```python
from build123d import *

# Parameters (mm, degrees)
SKETCH1_R           = 17.5
BOSS_EXTRUDE1_DEPTH = 0.5
SKETCH2_R           = 11.5
CUT_EXTRUDE1_DEPTH  = 0.5
SKETCH3_W           = 15
SKETCH3_H           = 8
CUT_EXTRUDE4_DEPTH  = 2.5
SKETCH4_R           = 16
SKETCH4_R_2         = 15.5
BOSS_EXTRUDE2_DEPTH = 4.5
SKETCH5_R           = 14.5
SKETCH5_R_2         = 14
BOSS_EXTRUDE3_DEPTH = 4.5
SKETCH6_R           = 17.5
SKETCH6_R_2         = 17
BOSS_EXTRUDE4_DEPTH = 4.5


with BuildPart() as part:
    # Sketch1 → Boss-Extrude1 (new body)
    with BuildSketch(Plane(origin=(0, 0, 0), x_dir=(1, 0, 0), z_dir=(0, 1, 0))):
        with Locations(Location((0, 0, 0), (0, 0, 270))):
            Circle(SKETCH1_R)
    extrude(amount=BOSS_EXTRUDE1_DEPTH)

    # Sketch2 → Cut-Extrude1 (cut)
    with BuildSketch(Plane(origin=(0, 0.5, 0), x_dir=(1, 0, 0), z_dir=(0, 1, 0))):
        with Locations(Location((2, 0, 0), (0, 0, 270))):
            Circle(SKETCH2_R)
    extrude(amount=-CUT_EXTRUDE1_DEPTH, mode=Mode.SUBTRACT)

    # Sketch3 → Cut-Extrude4 (cut)
    with BuildSketch(Plane(origin=(0, 0, 0), x_dir=(1, 0, 0), z_dir=(0, 1, 0))):
        with Locations((-5.5, 0)):
            Rectangle(SKETCH3_W, SKETCH3_H)
    extrude(amount=CUT_EXTRUDE4_DEPTH, mode=Mode.SUBTRACT)

    # Sketch4 → Boss-Extrude2 (add)
    with BuildSketch(Plane(origin=(0, 0, 0), x_dir=(1, 0, 0), z_dir=(0, 1, 0))):
        with Locations(Location((0, 0, 0), (0, 0, 270))):
            Circle(SKETCH4_R)
        with Locations(Location((0, 0, 0), (0, 0, 270))):
            Circle(SKETCH4_R_2, mode=Mode.SUBTRACT)
    extrude(amount=BOSS_EXTRUDE2_DEPTH)

    # Sketch5 → Boss-Extrude3 (add)
    with BuildSketch(Plane(origin=(0, 0.5, 0), x_dir=(1, 0, 0), z_dir=(0, 1, 0))):
        with Locations(Location((0, 0, 0), (0, 0, 270))):
            Circle(SKETCH5_R)
        with Locations(Location((0, 0, 0), (0, 0, 270))):
            Circle(SKETCH5_R_2, mode=Mode.SUBTRACT)
    extrude(amount=BOSS_EXTRUDE3_DEPTH)

    # Sketch6 → Boss-Extrude4 (add)
    with BuildSketch(Plane(origin=(0, 0.5, 0), x_dir=(1, 0, 0), z_dir=(0, 1, 0))):
        with Locations(Location((0, 0, 0), (0, 0, 270))):
            Circle(SKETCH6_R)
        with Locations(Location((0, 0, 0), (0, 0, 270))):
            Circle(SKETCH6_R_2, mode=Mode.SUBTRACT)
    extrude(amount=BOSS_EXTRUDE4_DEPTH)


solid = part.part
```
For this review, take the finished solid that the model builds, in its own axes (mm). A direction names the side the tool comes from. Give positions to 0.01 mm unless a question says otherwise; leave off trailing zeros. Loops run counter-clockwise (first coordinate to the right, second up) from the corner with the lowest first, then second, coordinate; pieces in that order, holes last. Notation, with made-up numbers: M 83,61.25 L 94,61.25 A16 cw 94,82.25 Z; hole C 57.5,-9.75 d6. An arc over 180 degrees is marked long. One line per item, written item: value. Start each with the question number.
Q1. Draft analysis for pull direction Z (two halves, no side actions). For faces 1 (the face through (-10.648, 2.465, -13.887)), 2 (the face through (-8, 0, 8)), 3 (the face through (-13.67, 2.72, -3.03)), state which applies: released by +Z, released by -Z, zero draft, split by the parting line, or undercut.
Q2. Add section B-B (z = 0). Give the boundary of the cut face in (x, y), and give its area (4 significant figures).
Q3. For L1, parallel to X at y = 3.6, z = -4.5; L2, parallel to X at y = 3.75, z = 1, list the stretches that pass through material, from the lowest coordinate up.
Q4. Add section A-A (y = 2.8). Give the boundary of the cut face in (x, z), and give its area (3 significant figures).
Q5. Add section C-C (x = -12). Give the boundary of the cut face in (y, z), and give its area (3 significant figures).
Q6. Clearance check with flat-ended pins moving along their axes: pin 1 Ø2 at (y, z) = (1, 1.5) entering from -X; pin 2 Ø1 at (y, z) = (2.5, -2.5) entering from -X; pin 3 Ø1.5 at (x, y) = (-8.5, 2) entering from -Z. State where each tip first meets the part, or that it passes through.
Q7. Machinability: for faces 4 (the face through (16.855, 2.718, -2.213)), 5 (the face through (13.49, 0.25, 0.45)), which of the approach directions +Z, -Z, +X, -X, +Y, -Y give a long, thin tool a straight path to every point of the face, cutting with its end or side? Answer none if there is none.
Reply:
1. face 1: split by the parting line
1. face 2: zero draft
1. face 3: undercut
2. outline: M -17.5,0 L -13,0 L -13,0.5 L -14,0.5 L -14,5 L -14.5,5 L -14.5,0.5 L -15.5,0.5 L -15.5,4.5 L -16,4.5 L -16,0.5 L -17,0.5 L -17,5 L -17.5,5 Z; M 13.5,0 L 17.5,0 L 17.5,5 L 17,5 L 17,0.5 L 16,0.5 L 16,4.5 L 15.5,4.5 L 15.5,0.5 L 14.5,0.5 L 14.5,5 L 14,5 L 14,0.5 L 13.5,0.5 Z
2. area: 17.25 mm²
3. L1: -16.91 to -16.39, -15.35 to -14.83, -13.78 to -13.26, 13.26 to 13.78, 14.83 to 15.35, 16.39 to 16.91
3. L2: -17.47 to -16.97, -15.97 to -15.47, -14.47 to -13.96, 13.96 to 14.47, 15.47 to 15.97, 16.97 to 17.47
4. outline: C 0,0 d35; C 0,0 d32; C 0,0 d29; hole C 0,0 d34; hole C 0,0 d31; hole C 0,0 d28
4. area: 148 mm²
5. outline: M 0,-12.74 L 5,-12.74 L 5,-12.04 L 0.5,-12.04 L 0.5,-10.58 L 4.5,-10.58 L 4.5,-9.81 L 0.5,-9.81 L 0.5,-8.14 L 5,-8.14 L 5,-7.21 L 0.5,-7.21 L 0.5,-4 L 0,-4 Z; M 0,4 L 0.5,4 L 0.5,7.21 L 5,7.21 L 5,8.14 L 0.5,8.14 L 0.5,9.81 L 4.5,9.81 L 4.5,10.58 L 0.5,10.58 L 0.5,12.04 L 5,12.04 L 5,12.74 L 0,12.74 Z
5. area: 29.5 mm²
6. pin 1: x = -17.49
6. pin 2: x = -17.39
6. pin 3: z = -15.69
7. face 4: +Y
7. face 5: +Y, -Y
